from build123d import *

# Parameters (mm, degrees)
F0_R     = 30
F1_DEPTH = 72
F2_SIZE  = 2
F3_SIZE2 = 3.464102
F3_SIZE  = 6
F4_W     = 15
F4_H     = 9
F5_DEPTH = 50


with BuildPart() as f1:
    # F0 (on Top) → F1 (new body, symmetric)
    with BuildSketch(Plane.XY):
        Circle(F0_R)
    extrude(amount=F1_DEPTH, both=True)

    # F2
    f2_edges = [f1.edges().sort_by_distance(p)[0] for p in [
        (-30, 0, 72),
    ]]
    chamfer(f2_edges, length=F2_SIZE)

    # F3
    f3_edges = [f1.edges().sort_by_distance(p)[0] for p in [
        (-30, 0, -72),
    ]]
    chamfer(f3_edges, length=F3_SIZE, length2=F3_SIZE2)

    # F4 (on Front) → F5 (cut, symmetric)
    with BuildSketch(Plane.XZ):
        with Locations((27.5, 60.5)):
            Rectangle(F4_W, F4_H)
    extrude(amount=F5_DEPTH, both=True, mode=Mode.SUBTRACT)


solid = f1.part
Could you check a few things on this model? Use its own coordinates, in mm. A direction names the side the tool comes from. Round coordinates to 2 decimals unless told otherwise and drop trailing zeros. Order: outer loops, then holes, each group sorted by start corner. A loop starts at its lowest first (then second) coordinate and runs counter-clockwise, first axis right, second up. Notation, with made-up numbers: M -11.75,-23 L 21.25,-23 A20 cw 21.25,-7 Z; hole C 31.5,-21 d4. An arc over 180 degrees is marked long. One line per item, written item: value.
(1) If we mould it in two halves opening along Z, with no side actions, what happens to faces 3 (the flat face through (24, 0, 56)), 4 (the flat face through (0, 0, -72)), 5 (the flat face through (0, 0, 72))? For each: released by +Z, released by -Z, zero draft, split by the parting line, or undercut.
Ans:
face 3: undercut
face 4: released by -Z
face 5: released by +Z
(2) Imagine slicing it at A-A (z = 47.5). Write out the boundary of the cut face in (x, y).
Ans:
outline: C 0,0 d60
(3) Which directions (+Z, -Z, +X, -X, +Y, -Y) give clear straight access to the entire face, cutting with the end or side of a thin tool? Please do faces 1 (the conical face through (25.47, 8.02, -71.71)), 2 (the flat face through (20, 0, 60)).
Ans:
face 1: -Z
face 2: +X, +Y, -Y
(4) I'm going to push flat-ended pins straight in: P1, Ø1, axis at x = 16, z = -18, coming from the -Y side; P2, Ø1.5, axis at y = 21, z = 5, coming from the +X side; P3, Ø2, axis at x = 9.5, z = 15.5, coming from the -Y side. Where does each tip first touch, or does it pass through?
Ans:
P1: stops at y = -25.69
P2: stops at x = 22.13
P3: stops at y = -28.77
(5) I need wall thicknesses on line 1 along Z through (x, y) = (21, -14); line 2 along X through (y, z) = (-14, -2.5); line 3 along X through (y, z) = (1, 21). Which ranges of each line are inside material? Lowest first, please. Write a range as from..to.
Ans:
line 1: z = -72..56, 65..72
line 2: x = -26.53..26.53
line 3: x = -29.98..29.98
